For this review, use the dimensioned drawing (mm, ordinates from the lowest corner) and the shaded views. A direction names the side the tool comes from. Coordinates: 2 decimals unless noted, no trailing zeros. Loops run counter-clockwise (first coordinate to the right, second up) from the corner with the lowest first, then second, coordinate; pieces in that order, holes last. Notation, with made-up numbers: M -4,-36 L 28,-36 A20 cw 28,-12 Z; hole C 30,50.25 d10. An arc over 180 degrees is marked long. Use CSV: the item, a comma, the result in double quotes. Start each with the question number.
1. Clearance check with flat-ended pins moving along their axes: P1, Ø12, axis at x = 22.5, z = 28, coming from the -Y side; P2, Ø4, axis at y = 4.5, z = 26.5, coming from the +X side (1 decimal); P3, Ø1, axis at y = 7, z = 15.5, coming from the +X side. State where each tip first meets the part, or that it passes through.
2. For L1, parallel to Z at x = 17.5, y = 2.65; L2, parallel to Y at x = 26, z = 12; L3, parallel to X at y = 7.5, z = 27.5, list the stretches that pass through material, from the lowest coordinate up.
3. Add section A-A, the plane z = 17.5. Write out the cut boundary in (x, y).
4. Add section C-C, the plane y = 6.75. Write out the cut boundary in (x, z).
5. Add section B-B, the plane x = 17.5. Write out the cut boundary in (y, z).
6. Tool access review of the marked faces 1 and 2: name each direction out of +Z, -Z, +X, -X, +Y, -Y from which nothing blocks a thin tool from reaching the whole face with its end or side.
7. Add section D-D, the plane x = 28. Write out the cut boundary in (y, z).
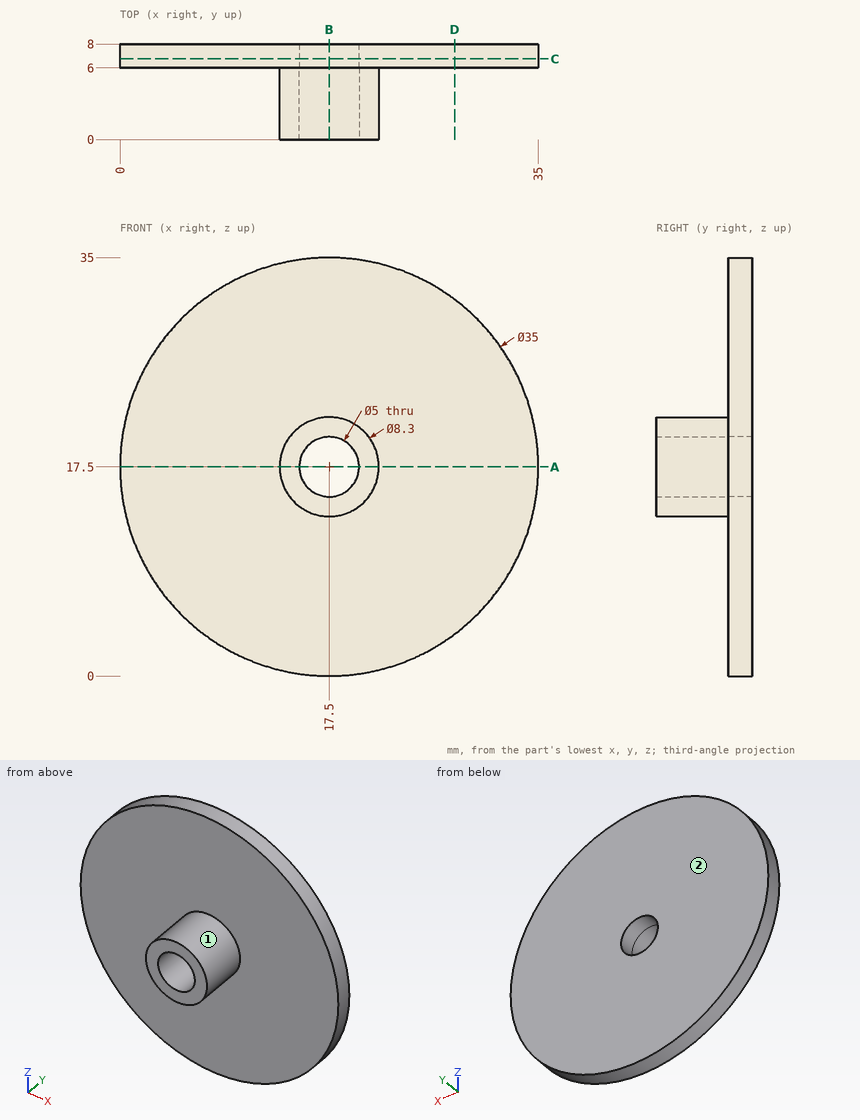
Computed:
1,P1,"stops at y = 6"
1,P2,"stops at x = 33.2"
1,P3,"stops at x = 34.94"
2,L1,"z = 13.35 to 15, 20 to 21.65"
2,L2,"y = 6 to 8"
2,L3,"x = 3.14 to 31.86"
3,outline,"M 0,6 L 13.35,6 L 13.35,0 L 15,0 L 15,8 L 0,8 Z; M 20,0 L 21.65,0 L 21.65,6 L 35,6 L 35,8 L 20,8 Z"
4,outline,"C 17.5,17.5 d35; hole C 17.5,17.5 d5"
5,outline,"M 0,13.35 L 6,13.35 L 6,0 L 8,0 L 8,15 L 0,15 Z; M 0,20 L 8,20 L 8,35 L 6,35 L 6,21.65 L 0,21.65 Z"
6,face 1,"-Y"
6,face 2,"+Z, -Z, +X, -X, +Y"
7,outline,"M 6,3.5 L 8,3.5 L 8,31.5 L 6,31.5 Z"
